Model file for the job. Use its own axes, mm. A direction names the side the tool comes from. Round coordinates to 2 decimals unless told otherwise and drop trailing zeros. Order: outer loops, then holes, each group sorted by start corner. A loop starts at its lowest first (then second) coordinate and runs counter-clockwise, first axis right, second up. Notation, with made-up numbers: (27.25, 21.5) -> (82.25, 21.5) arc R18 ccw to (82.25, 49.5) -> close; hole circle Ø5 at (26.25, -12.5). An arc over 180 degrees is marked (long way). Put each result on its own line as item: value. Start each with the question number.
Q1. Probe L1, parallel to X at y = 12.75, z = -7; L2, parallel to X at y = 9, z = -14; L3, parallel to Z at x = 22.5, y = 8.5. List the from-to ranges inside material, lowest first.
Q2. 3-axis set-ups, long thin cutter, end or side, ignore diameter. For faces 4 (the face through (22.6, 11.8, 14.2)), 5 (the face through (-22, 9, -14)), 6 (the face through (30, 6, 14.5)): which of +Z, -Z, +X, -X, +Y, -Y reach the whole face in a straight line?
Q3. Cut at D-D, the plane x = -20. List the corners of the cut face in (y, z).
Q4. Pull direction Z, two halves, no side cores. Call faces 1 (the face through (0.1, 2.6, -17.5)), 2 (the face through (6, 9, 17)), 3 (the face through (15, 9, 15.5)): released by +Z, released by -Z, zero draft, split by the parting line, or undercut.
Q5. Cut at A-A, the plane y = 14. State how many separate pieces and enclosed holes the cut face has, and give its area (3 significant figures).
Q6. Cut at C-C, the plane y = 4.25. List the corners of the cut face in (x, z), and give its area (3 significant figures).
Q7. Cut at B-B, the plane z = -7. List the corners of the cut face in (x, y), and give its area (3 significant figures).
Q8. Flat gauge pins, fed straight in: P1, Ø1, axis at x = 14, z = -0.5, coming from the +Y side; P2, Ø8, axis at x = 1.5, y = 14, coming from the -Z side; P3, Ø5, axis at x = 32.5, y = 8.5, coming from the -Z side. Where does each tip first touch, or does it go through?
from build123d import *

# Parameters (mm, degrees)
SKETCH1_W           = 50
SKETCH1_H           = 35
BOSS_EXTRUDE1_DEPTH = 3
BOSS_EXTRUDE2_DEPTH = 12.7
CHAMFER1_SIZE       = 3
SKETCH3_R           = 0.9
CUT_EXTRUDE1_DEPTH  = 8
SKETCH4_R           = 0.9
CUT_EXTRUDE2_DEPTH  = 8
SKETCH5_R           = 0.9
CUT_EXTRUDE3_DEPTH  = 8
SKETCH6_W           = 3
SKETCH6_H           = 15.7
BOSS_EXTRUDE3_DEPTH = 10
SKETCH7_W           = 3
SKETCH7_H           = 15.7
BOSS_EXTRUDE4_DEPTH = 10
SKETCH8_R           = 1.55
CUT_EXTRUDE4_DEPTH  = 10


with BuildPart() as part:
    # Sketch1 → Boss-Extrude1 (new body)
    with BuildSketch(Plane(origin=(0, 0, 0), x_dir=(1, 0, 0), z_dir=(0, 1, 0))):
        Rectangle(SKETCH1_W, SKETCH1_H)
    extrude(amount=BOSS_EXTRUDE1_DEPTH)

    # Sketch2 → Boss-Extrude2 (add)
    with BuildSketch(Plane(origin=(0, 3, 0), x_dir=(1, 0, 0), z_dir=(0, 1, 0))):
        Polygon((25, 17.5), (22, 17.5), (22, 11.5), (6.5, 11.5), (6.5, 2.5), (22, 2.5), (22, -15.5), (11, -15.5), (11, -17.5), (22, -17.5), (25, -17.5), (25, 2.5), (25, 11.5), align=None)
        Polygon((-17.5, 11.5), (-22, 11.5), (-22, 17.5), (-25, 17.5), (-25, 11.5), (-25, 2.5), (-25, -17.5), (-22, -17.5), (6, -17.5), (6, -15.5), (-22, -15.5), (-22, 2.5), (-17.5, 2.5), align=None)
    extrude(amount=BOSS_EXTRUDE2_DEPTH)

    # Chamfer1
    chamfer1_edges = [part.edges().sort_by_distance(p)[0] for p in [
        (22, 9.35, 15.5),
        (-22, 9.35, 15.5),
    ]]
    chamfer(chamfer1_edges, length=CHAMFER1_SIZE)

    # Sketch3 → Cut-Extrude1 (cut)
    with BuildSketch(Plane(origin=(0, 15.7, 0), x_dir=(1, 0, 0), z_dir=(0, 1, 0))):
        with Locations(Location((-22.6, -15.1, 0), (0, 0, 270))):
            Circle(SKETCH3_R)
        with Locations(Location((22.6, -15.1, 0), (0, 0, 270))):
            Circle(SKETCH3_R)
        with Locations(Location((22.6, 7, 0), (0, 0, 270))):
            Circle(SKETCH3_R)
    extrude(amount=-CUT_EXTRUDE1_DEPTH, mode=Mode.SUBTRACT)

    # Sketch4 → Cut-Extrude2 (cut)
    with BuildSketch(Plane(origin=(0, 15.7, 0), x_dir=(1, 0, 0), z_dir=(0, 1, 0))):
        with Locations(Location((-22.6, 7, 0), (0, 0, 270))):
            Circle(SKETCH4_R)
    extrude(amount=-CUT_EXTRUDE2_DEPTH, mode=Mode.SUBTRACT)

    # Sketch5 → Cut-Extrude3 (cut)
    with BuildSketch(Plane(origin=(0, 0, -11.5), x_dir=(-1, 0, 0), z_dir=(0, 0, -1))):
        with Locations((20, 9.35)):
            Circle(SKETCH5_R)
        with Locations((-9, 9.35)):
            Circle(SKETCH5_R)
    extrude(amount=-CUT_EXTRUDE3_DEPTH, mode=Mode.SUBTRACT)

    # Sketch6 → Boss-Extrude3 (add)
    with BuildSketch(Plane.ZY.offset(25)):
        with Locations((16, 7.85)):
            Rectangle(SKETCH6_W, SKETCH6_H)
    extrude(amount=BOSS_EXTRUDE3_DEPTH)

    # Sketch7 → Boss-Extrude4 (add)
    with BuildSketch(Plane(origin=(25, 0, 0), x_dir=(0, 0, -1), z_dir=(1, 0, 0))):
        with Locations((-16, 7.85)):
            Rectangle(SKETCH7_W, SKETCH7_H)
    extrude(amount=BOSS_EXTRUDE4_DEPTH)

    # Sketch8 → Cut-Extrude4 (cut)
    with BuildSketch(Plane(origin=(0, 0, 14.5), x_dir=(-1, 0, 0), z_dir=(0, 0, -1))):
        with Locations(Location((30, 7.85, 0), (0, 0, 90))):
            Circle(SKETCH8_R)
        with Locations(Location((-30, 7.85, 0), (0, 0, 90))):
            Circle(SKETCH8_R)
    extrude(amount=-CUT_EXTRUDE4_DEPTH, mode=Mode.SUBTRACT)


solid = part.part
Ans:
1. L1: x = -25 to -23.5, -21.7 to -17.5, 6.5 to 21.7, 23.5 to 25
1. L2: x = -25 to -22, 22 to 25
1. L3: z = -17.5 to -7.89, -6.11 to 14.21, 15.99 to 17.5
2. face 4: +Y
2. face 5: -Z, +Y
2. face 6: -Z, +X, +Y, -Y
3. outline: (0, -17.5) -> (3, -17.5) -> (3, -11.5) -> (8.45, -11.5) -> (8.45, -3.5) -> (10.25, -3.5) -> (10.25, -11.5) -> (15.7, -11.5) -> (15.7, -2.5) -> (3, -2.5) -> (3, 14.5) -> (15.7, 14.5) -> (15.7, 17.5) -> (0, 17.5) -> close
4. face 1: released by -Z
4. face 2: zero draft
4. face 3: undercut
5. separate pieces: 2
5. enclosed holes: 4
5. area: 527 mm^2
6. outline: (-35, 14.5) -> (-25, 14.5) -> (-25, -17.5) -> (-22, -17.5) -> (-22, -11.5) -> (-17.5, -11.5) -> (-17.5, -2.5) -> (-22, -2.5) -> (-22, 12.5) -> (-19, 15.5) -> (6, 15.5) -> (6, 17.5) -> (-35, 17.5) -> close; (6.5, -11.5) -> (22, -11.5) -> (22, -17.5) -> (25, -17.5) -> (25, 14.5) -> (35, 14.5) -> (35, 17.5) -> (11, 17.5) -> (11, 15.5) -> (19, 15.5) -> (22, 12.5) -> (22, -2.5) -> (6.5, -2.5) -> close
6. area: 537 mm^2
7. outline: (-25, 0) -> (25, 0) -> (25, 15.7) -> (23.5, 15.7) -> (23.5, 7.7) -> (21.7, 7.7) -> (21.7, 15.7) -> (6.5, 15.7) -> (6.5, 3) -> (-17.5, 3) -> (-17.5, 15.7) -> (-21.7, 15.7) -> (-21.7, 7.7) -> (-23.5, 7.7) -> (-23.5, 15.7) -> (-25, 15.7) -> close; hole circle Ø1.8 at (-20, 9.35); hole circle Ø1.8 at (9, 9.35)
7. area: 446 mm^2
8. P1: stops at y = 3
8. P2: stops at z = 15.5
8. P3: stops at z = 14.5
